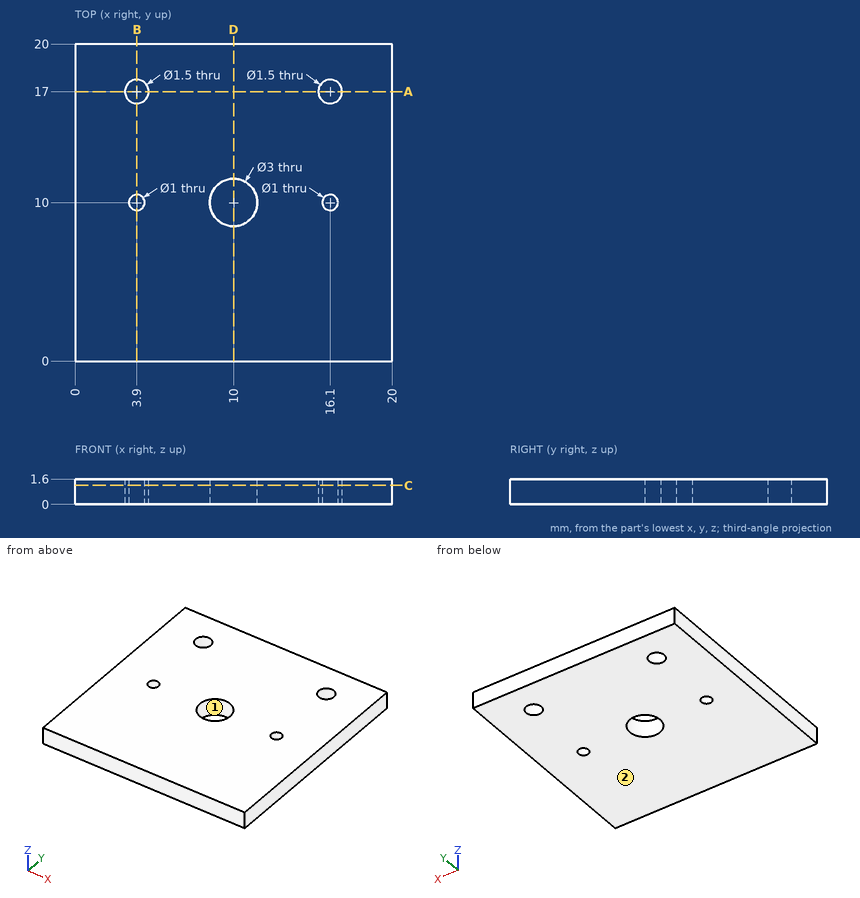
Job drawing, mm, ordinate dimensions from the low corner. One solid piece. Give positions to 0.01 mm unless a question says otherwise; leave off trailing zeros. Loops run counter-clockwise (first coordinate to the right, second up) from the corner with the lowest first, then second, coordinate; pieces in that order, holes last. Notation, with made-up numbers: M 53,45 L 95,45 A13 cw 95,60 Z; hole C 10,-34 d4. An arc over 180 degrees is marked long. Use one line per item in the form item = value.
Item 1: Two-plate mould, pull along X, no slides. Class the marked faces 1 and 2: released by +X, released by -X, zero draft, split by the parting line, or undercut.
Filled in:
face_1 = undercut
face_2 = zero draft
Item 2: Slice it at D-D on x = 10. List the corners of the cut face in (y, z).
Filled in:
outline = M 0,0 L 8.5,0 L 8.5,1.6 L 0,1.6 Z; M 11.5,0 L 20,0 L 20,1.6 L 11.5,1.6 Z
Item 3: Slice it at C-C on z = 1.2. List the corners of the cut face in (x, y), and give its area (3 significant figures).
Filled in:
outline = M 0,0 L 20,0 L 20,20 L 0,20 Z; hole C 3.9,17 d1.5; hole C 3.9,10 d1; hole C 10,10 d3; hole C 16.1,17 d1.5; hole C 16.1,10 d1
area = 388 mm^2
Item 4: Flat gauge pin, fed straight in: pin 1 Ø0.9 at (x, y) = (3.9, 17) entering from -Z. Where does the tip first touch, or does it go through?
Filled in:
pin_1 = through
Item 5: Slice it at A-A on y = 17. List the corners of the cut face in (x, z), and give its area (3 significant figures).
Filled in:
outline = M 0,0 L 3.15,0 L 3.15,1.6 L 0,1.6 Z; M 4.65,0 L 15.35,0 L 15.35,1.6 L 4.65,1.6 Z; M 16.85,0 L 20,0 L 20,1.6 L 16.85,1.6 Z
area = 27.2 mm^2
Item 6: Slice it at B-B on x = 3.9. List the corners of the cut face in (y, z), and give its area (3 significant figures).
Filled in:
outline = M 0,0 L 9.5,0 L 9.5,1.6 L 0,1.6 Z; M 10.5,0 L 16.25,0 L 16.25,1.6 L 10.5,1.6 Z; M 17.75,0 L 20,0 L 20,1.6 L 17.75,1.6 Z
area = 28.0 mm^2
Item 7: Drill centre lines: L1, parallel to Y at x = 3.9, z = 0.7; L2, parallel to Y at x = 10, z = 0.7; L3, parallel to X at y = 8.75, z = 0.5. Where is each one in solid material? Low to high.
Filled in:
L1 = 0 to 9.5, 10.5 to 16.25, 17.75 to 20
L2 = 0 to 8.5, 11.5 to 20
L3 = 0 to 9.17, 10.83 to 20
